from build123d import *

# Parameters (mm, degrees)
CHAMFER1_SIZE      = 0.5
SKETCH3_R          = 1.5
CUT_EXTRUDE1_DEPTH = 76


with BuildPart() as part:
    # Sketch2 → Revolve1 (revolve)
    with BuildSketch(Plane(origin=(0, 0, 0), x_dir=(1, 0, 0), z_dir=(0, 1, 0))):
        Polygon((-34, 1), (-34, 2.25), (-31, 5.25), (31, 5.25), (31, 12.5), (41, 12.5), (41, 1), (39, 0), (-32, 0), align=None)
    revolve(axis=Axis((-32, 0, 0), (1, 0, 0)))

    # Chamfer1
    chamfer1_edges = [part.edges().sort_by_distance(p)[0] for p in [
        (41, 0, 12.5),
        (31, 0, 12.5),
    ]]
    chamfer(chamfer1_edges, length=CHAMFER1_SIZE)

    # Sketch3 → Cut-Extrude1 (cut, through all)
    with BuildSketch(Plane(origin=(41, 0, 0), x_dir=(0, 0, -1), z_dir=(1, 0, 0))):
        with Locations((0, 7)):
            Circle(SKETCH3_R)
        with Locations((4.949747468, 4.949747468)):
            Circle(SKETCH3_R)
        with Locations((7, 0)):
            Circle(SKETCH3_R)
        with Locations((4.949747468, -4.949747468)):
            Circle(SKETCH3_R)
        with Locations((0, -7)):
            Circle(SKETCH3_R)
        with Locations((-4.949747468, -4.949747468)):
            Circle(SKETCH3_R)
        with Locations((-7, 0)):
            Circle(SKETCH3_R)
        with Locations((-4.949747468, 4.949747468)):
            Circle(SKETCH3_R)
    extrude(amount=-CUT_EXTRUDE1_DEPTH, mode=Mode.SUBTRACT)


solid = part.part
Read the model definition and answer for the solid it produces. Units are mm, in the model's axes. A direction names the side the tool comes from. Coordinates: 2 decimals unless noted, no trailing zeros. Order: outer loops, then holes, each group sorted by start corner. A loop starts at its lowest first (then second) coordinate and runs counter-clockwise, first axis right, second up. Notation, with made-up numbers: M 13.25,52 L 31.25,52 A23 cw 31.25,69 Z; hole C 68.5,-30.75 d1. An arc over 180 degrees is marked long. Put each result on its own line as item: value. Start each with the question number.
Item 1: Section A-A, the plane x = 26 is taken. Determine the outline of the cut face in (y, z), plus the area to 3 significant figures.
Item 2: Given pin 1 Ø4 at (x, y) = (25, -1) entering from -Z; pin 2 Ø2.5 at (y, z) = (4.95, -4.95) entering from +X; pin 3 Ø1.5 at (y, z) = (-5.5, 9) entering from -X; pin 4 Ø6 at (x, y) = (-14.5, 4.5) entering from +Z, each flat-ended and moving along its own axis, determine where each tip first touches the part or whether it passes through.
Item 3: The mould has two halves that part along Z. Classify faces 3 (the face through (-33.8, -2.4, 0.5)), 4 (the face through (41, -2, 0)), 5 (the face through (36.07, 0.07, 8.5)): +Z half, -Z half, draft (parallel to the pull), parting line (faces both ways), or undercut.
Item 4: For faces 1 (the face through (36.07, 0.07, -5.5)), 2 (the face through (0.4, 1.6, -5)), determine the directions among +Z, -Z, +X, -X, +Y, -Y from which every point of the face is accessible in a straight line to the end or side of a thin tool.
Item 5: Consider probe 1 along Y at (x, z) = (36, 0); probe 2 along X at (y, z) = (4.5, -7); probe 3 along Z at (x, y) = (-14, 4.75). Determine where each line is inside the solid, lowest interval first. Write a range as [from, to].
Computed:
1. outline: C 0,0 d10.5
1. area: 86.6 mm2
2. pin 1: stops at z = -5.25
2. pin 2: passes through
2. pin 3: stops at x = 31
2. pin 4: stops at z = 5.03
3. face 3: parting line
3. face 4: draft
3. face 5: undercut
4. face 1: +X, -X
4. face 2: -X
5. probe 1: y = [-12.5, -8.5], [-5.5, 5.5], [8.5, 12.5]
5. probe 2: x = [31, 41]
5. probe 3: z = [-2.24, 2.24]
